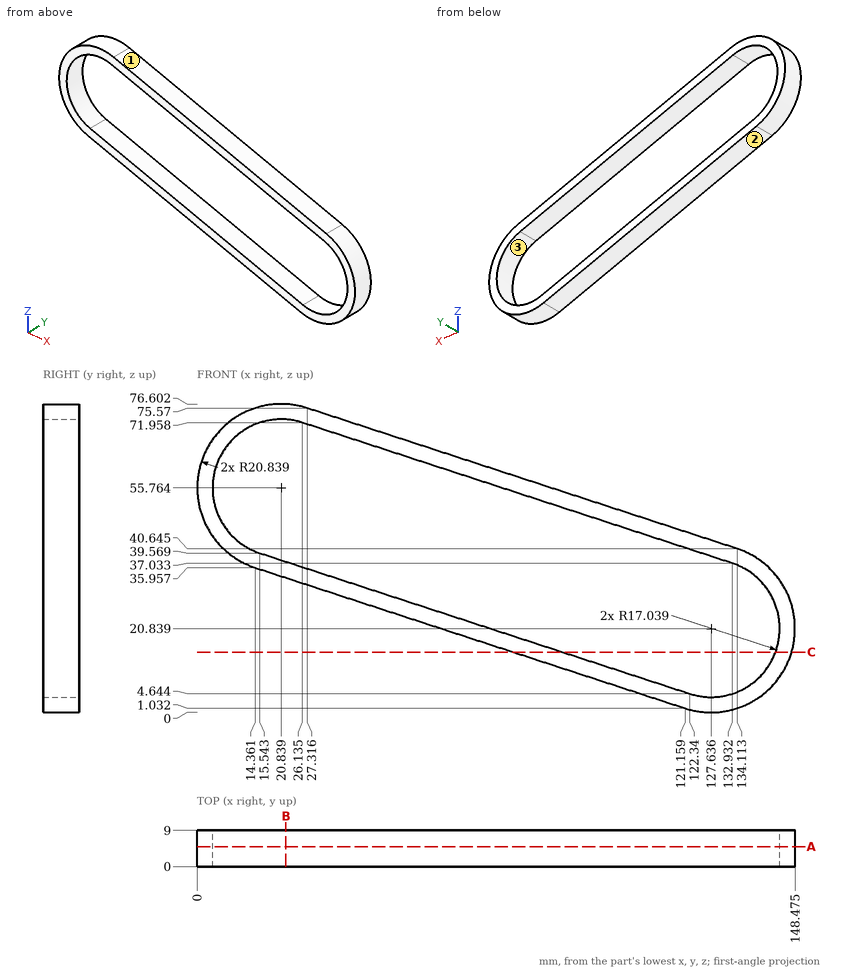
Geometry: see drawing. Coordinates: mm, zero at the bounding-box minimum. Round coordinates to 2 decimals unless told otherwise and drop trailing zeros. Write each loop counter-clockwise with the first axis right and the second up, starting at its lowest first coordinate (ties: lowest second). Pieces come first, ordered by that corner, then holes.
Item 1: Section query A-A (y = 5). Return loops of the section in (x, z) (1 decimal).
Item 2: Mould query, pull axis X, two halves, no side actions, for the marked faces 1, 2 and 3. Classes: +X half, -X half, draft (parallel to the pull), parting line (faces both ways), or undercut.
Item 3: Material intervals for L1, parallel to Z at x = 86, y = 4; L2, parallel to Z at x = 46, y = 4.5, sorted ascending.
Item 4: Section query C-C (z = 15). Return loops of the section in (x, y).
Item 5: Section query B-B (x = 22). Return loops of the section in (y, z).
Item 6: Pin query (flat end, axial travel): P1, Ø4, axis at x = 71, y = 4.5, coming from the -Z side; P2, Ø1.5, axis at y = 4.5, z = 33, coming from the +X side; P3, Ø1.5, axis at x = 109.5, y = 4, coming from the +Z side. Return the tip coordinate at first contact, or that it passes through.
Completed:
1. outline: (14.4, 36) - (121.2, 1) arc R20.8 ccw to (134.1, 40.6) - (27.3, 75.6) arc R20.8 ccw to start; hole (15.5, 39.6) - (122.3, 4.6) arc R17 ccw to (132.9, 37) - (26.1, 72) arc R17 ccw to start
2. face 1: +X half
2. face 2: -X half
2. face 3: undercut
3. L1: z = 12.53 to 16.53, 52.38 to 56.38
3. L2: z = 25.61 to 29.61, 65.46 to 69.46
4. outline: (78.45, 0) - (90.67, 0) - (90.67, 9) - (78.45, 9) - close; (143.64, 0) - (147.64, 0) - (147.64, 9) - (143.64, 9) - close
5. outline: (0, 33.46) - (9, 33.46) - (9, 37.46) - (0, 37.46) - close; (0, 72.76) - (9, 72.76) - (9, 76.57) - (0, 76.57) - close
6. P1: stops at z = 16.78
6. P2: stops at x = 145.07
6. P3: stops at z = 48.94
